from build123d import *

# Parameters (mm, degrees)
RESSALTO_EXTRUS_O2_DEPTH = 6.5


with BuildPart() as part:
    # Esboço1 → Ressalto-extrusão2 (new body)
    with BuildSketch(Plane(origin=(0, 0, 0), x_dir=(1, 0, 0), z_dir=(0, 1, 0))):
        with BuildLine():
            Line((-1.3, -1.64924225), (-1.3, 1.64924225))
            ThreePointArc((-1.3, 1.64924225), (-2.1, 0), (-1.3, -1.64924225))
        make_face()
        with BuildLine():
            Line((-1.3, 1.64924225), (-1.3, 2.25166605))
            ThreePointArc((-1.3, 2.25166605), (-2.6, 0), (-1.3, -2.25166605))
            Line((-1.3, -2.25166605), (-1.3, -1.64924225))
            ThreePointArc((-1.3, -1.64924225), (-2.1, 0), (-1.3, 1.64924225))
        make_face()
        with BuildLine():
            Line((0, 2.1), (0, 2.6))
            ThreePointArc((0, 2.6), (-0.672929517, 2.511407148), (-1.3, 2.25166605))
            Line((-1.3, 2.25166605), (-1.3, 1.64924225))
            ThreePointArc((-1.3, 1.64924225), (-0.687964852, 1.984112991), (0, 2.1))
        make_face()
        with BuildLine():
            Line((0, -2.6), (0, -2.1))
            ThreePointArc((0, -2.1), (-0.687964852, -1.984112991), (-1.3, -1.64924225))
            Line((-1.3, -1.64924225), (-1.3, -2.25166605))
            ThreePointArc((-1.3, -2.25166605), (-0.672929517, -2.511407148), (0, -2.6))
        make_face()
        with BuildLine():
            ThreePointArc((1.3, 2.25166605), (0.672929517, 2.511407148), (0, 2.6))
            Line((0, 2.6), (0, 2.1))
            ThreePointArc((0, 2.1), (0.687964852, 1.984112991), (1.3, 1.64924225))
            Line((1.3, 1.64924225), (1.3, 2.25166605))
        make_face()
        with BuildLine():
            ThreePointArc((1.3, -1.64924225), (0.687964852, -1.984112991), (0, -2.1))
            Line((0, -2.1), (0, -2.6))
            ThreePointArc((0, -2.6), (0.672929517, -2.511407148), (1.3, -2.25166605))
            Line((1.3, -2.25166605), (1.3, -1.64924225))
        make_face()
        with BuildLine():
            ThreePointArc((2.6, 0), (2.25166605, 1.3), (1.3, 2.25166605))
            Line((1.3, 2.25166605), (1.3, 1.64924225))
            ThreePointArc((1.3, 1.64924225), (1.889444363, 0.916515139), (2.1, 0))
            ThreePointArc((2.1, 0), (1.889444363, -0.916515139), (1.3, -1.64924225))
            Line((1.3, -1.64924225), (1.3, -2.25166605))
            ThreePointArc((1.3, -2.25166605), (2.25166605, -1.3), (2.6, 0))
        make_face()
        with BuildLine():
            ThreePointArc((2.1, 0), (1.889444363, 0.916515139), (1.3, 1.64924225))
            Line((1.3, 1.64924225), (1.3, -1.64924225))
            ThreePointArc((1.3, -1.64924225), (1.889444363, -0.916515139), (2.1, 0))
        make_face()
    extrude(amount=RESSALTO_EXTRUS_O2_DEPTH)


solid = part.part
Could you check a few things on this model? Use its own coordinates, in mm. A direction names the side the tool comes from. Give positions to 0.01 mm unless a question says otherwise; leave off trailing zeros. Loops run counter-clockwise (first coordinate to the right, second up) from the corner with the lowest first, then second, coordinate; pieces in that order, holes last. Notation, with made-up numbers: (27.25, 26) -> (31.25, 26) arc R15 cw to (31.25, 38) -> close; hole circle Ø9 at (14, 78.5). An arc over 180 degrees is marked (long way). Return JSON: item names as keys, results as strings.
Item 1: If we section it at B-B on z = 1.9: List the corners of the cut face in (x, y) for me, plus the area to 3 significant figures.
Geometry results:
{"outline": "(-1.77, 0) -> (-0.89, 0) -> (-0.89, 6.5) -> (-1.77, 6.5) -> close; (0.89, 0) -> (1.77, 0) -> (1.77, 6.5) -> (0.89, 6.5) -> close", "area": "11.4 mm²"}
Item 2: Which directions (+Z, -Z, +X, -X, +Y, -Y) give clear straight access to the entire face, cutting with the end or side of a thin tool? Please do faces 3 (the flat face through (1.3, 3, 0)), 4 (the flat face through (2, 6.5, 0)).
Geometry results:
{"face 3": "+Y, -Y", "face 4": "+Z, -Z, +X, -X, +Y"}
Item 3: I need wall thicknesses on L1, parallel to X at y = 5, z = 1.9; L2, parallel to X at y = 1.5, z = -0.25; L3, parallel to Z at x = -1, y = 3.5. Which ranges of each line are inside material? Lowest first, please. Write a range as from..to.
Geometry results:
{"L1": "x = -1.77..-0.89, 0.89..1.77", "L2": "x = -2.59..-1.3, 1.3..2.59", "L3": "z = -2.4..-1.85, 1.85..2.4"}
Item 4: If we section it at D-D on x = 1.8: List the corners of the cut face in (y, z) for me, plus the area to 3 significant figures.
Geometry results:
{"outline": "(0, -1.88) -> (6.5, -1.88) -> (6.5, 1.88) -> (0, 1.88) -> close", "area": "24.4 mm²"}
Item 5: We'd pull the mould along Z, two halves only. Please class faces 1 (the flat face through (2, 0, 0)), 2 (the flat face through (-1.3, 3, 0)): +Z half, -Z half, draft (parallel to the pull), parting line (faces both ways), or undercut.
Geometry results:
{"face 1": "draft", "face 2": "undercut"}
Item 6: If we section it at A-A on y = 4: List the corners of the cut face in (x, z) for me.
Geometry results:
{"outline": "circle Ø5.2 at (0, 0); hole (-1.3, -1.65) arc R2.1 ccw to (1.3, -1.65) -> (1.3, 1.65) arc R2.1 ccw to (-1.3, 1.65) -> close"}
Item 7: I'm going to push a flat-ended pin straight in: pin 1 (1 mm diameter, centred on x = 2, y = 2.5, fed in from -Z). Where does the tip first touch, or does it pass through?
Geometry results:
{"pin 1": "stops at z = -2.12"}
Item 8: If we section it at C-C on x = 1.1: List the corners of the cut face in (y, z) for me.
Geometry results:
{"outline": "(0, -2.36) -> (6.5, -2.36) -> (6.5, -1.79) -> (0, -1.79) -> close; (0, 1.79) -> (6.5, 1.79) -> (6.5, 2.36) -> (0, 2.36) -> close"}
